Could you check a few things on this model? Use its own coordinates, in mm. A direction names the side the tool comes from. Coordinates: 2 decimals unless noted, no trailing zeros. Write each loop counter-clockwise with the first axis right and the second up, starting at its lowest first coordinate (ties: lowest second). Pieces come first, ordered by that corner, then holes. Notation, with made-up numbers: (-1, 81) - (41, 81) arc R26 cw to (41, 95) - close; hole circle Ø1 at (6, 55). An arc over 180 degrees is marked (long way). Answer as a JSON object with one key per item and string values. Group by question number.
1) If we section it at B-B (y = 145.5): Write out the boundary of the cut face in (x, z).
2) We'd pull the mould along Z, two halves only. Please class faces 3 (the cylindrical face through (-17.5, 98.6, -40.07)), 4 (the flat face through (0, 99, -50)), 5 (the flat face through (25, 99, -46)): released by +Z, released by -Z, zero draft, split by the parting line, or undercut.
3) Will this pin go through, and if not, where does the flat tip stop? pin 1 Ø8 at (y, z) = (60, -28) entering from +X.
4) Please list where these lines run through material, in increasing order: line 1 along Z through (x, y) = (7, 168.5); line 2 along X through (y, z) = (24.5, -26.5); line 3 along Z through (x, y) = (-17.5, 151).
5) If we section it at A-A (x = 17.5): Write out the boundary of the cut face in (y, z).
6) If we section it at C-C (z = -5): Write out the boundary of the cut face in (x, y), plus the area to 3 significant figures.
7) On a 3-axis mill with a long thin cutter (end or side, diameter ignored), from which of +Z, -Z, +X, -X, +Y, -Y can I reach the whole of each face in a straight line? I mean faces 1 (the flat face through (-20, 0, -3)), 2 (the cylindrical face through (-17.57, 98.6, 40)). Say none if no direction works.
```python
from build123d import *

# Parameters (mm, degrees)
F1_DEPTH = 200


with BuildPart() as f1:
    # F0 (on Front) → F1 (new body)
    with BuildSketch(Plane.XZ):
        with BuildLine():
            Line((25, 41.5), (25, 50))
            Line((25, 50), (-25, 50))
            Line((-25, 50), (-25, -50))
            Line((-25, -50), (25, -50))
            Line((25, -50), (25, -41.5))
            Line((25, -41.5), (-14, -41.5))
            ThreePointArc((-14, -41.5), (-17.535534, -40.035534), (-19, -36.5))
            Line((-19, -36.5), (-19, 36.5))
            ThreePointArc((-19, 36.5), (-17.535534, 40.035534), (-14, 41.5))
            Line((-14, 41.5), (25, 41.5))
        make_face()
    extrude(amount=-F1_DEPTH)


solid = f1.part
```
Here are the results:
{
 "1": {"outline": "(-25, -50) - (25, -50) - (25, -41.5) - (-14, -41.5) arc R5 cw to (-19, -36.5) - (-19, 36.5) arc R5 cw to (-14, 41.5) - (25, 41.5) - (25, 50) - (-25, 50) - close"},
 "2": {"face 3": "undercut", "face 4": "released by -Z", "face 5": "zero draft"},
 "3": {"pin 1": "stops at x = -19"},
 "4": {"line 1": "z = -50 to -41.5, 41.5 to 50", "line 2": "x = -25 to -19", "line 3": "z = -50 to -40.07, 40.07 to 50"},
 "5": {"outline": "(0, -50) - (200, -50) - (200, -41.5) - (0, -41.5) - close; (0, 41.5) - (200, 41.5) - (200, 50) - (0, 50) - close"},
 "6": {"outline": "(-25, 0) - (-19, 0) - (-19, 200) - (-25, 200) - close", "area": "1,200 mm²"},
 "7": {"face 1": "+Z, -Z, +X, -X, -Y", "face 2": "+X, +Y, -Y"}
}
